from build123d import *

# Parameters (mm, degrees)
SKETCH1_R           = 12.5
BOSS_EXTRUDE1_DEPTH = 17
SKETCH2_R           = 20
BOSS_EXTRUDE2_DEPTH = 26.425
SKETCH3_R           = 12.7
BOSS_EXTRUDE3_DEPTH = 31.75
SKETCH8_W           = 6.35
SKETCH8_H           = 3.175
BOSS_EXTRUDE8_DEPTH = 31.75
SKETCH4_R           = 20
BOSS_EXTRUDE4_DEPTH = 171.45
SKETCH5_R           = 9.525
BOSS_EXTRUDE5_DEPTH = 31.75
SKETCH9_W           = 4.7625
SKETCH9_H           = 2.38125
BOSS_EXTRUDE9_DEPTH = 31.75
SKETCH6_R           = 20
BOSS_EXTRUDE6_DEPTH = 26.425
SKETCH7_R           = 12.5
BOSS_EXTRUDE7_DEPTH = 17


with BuildPart() as part:
    # Sketch1 → Boss-Extrude1 (new body)
    with BuildSketch(Plane(origin=(0, 0, 0), x_dir=(1, 0, 0), z_dir=(0, 1, 0))):
        with Locations(Location((0, 0, 0), (0, 0, 270))):
            Circle(SKETCH1_R)
    extrude(amount=BOSS_EXTRUDE1_DEPTH)

    # Sketch2 → Boss-Extrude2 (add)
    with BuildSketch(Plane(origin=(0, 17, 0), x_dir=(1, 0, 0), z_dir=(0, 1, 0))):
        with Locations(Location((0, 0, 0), (0, 0, 270))):
            Circle(SKETCH2_R)
    extrude(amount=BOSS_EXTRUDE2_DEPTH)

    # Sketch3 → Boss-Extrude3 (add)
    with BuildSketch(Plane(origin=(0, 43.425, 0), x_dir=(1, 0, 0), z_dir=(0, 1, 0))):
        with Locations(Location((0, 0, 0), (0, 0, 270))):
            Circle(SKETCH3_R)
    extrude(amount=BOSS_EXTRUDE3_DEPTH)

    # Sketch8 → Boss-Extrude8 (add)
    with BuildSketch(Plane(origin=(0, 75.175, 0), x_dir=(1, 0, 0), z_dir=(0, 1, 0))):
        with Locations((0, 13.884222124)):
            Rectangle(SKETCH8_W, SKETCH8_H)
    extrude(amount=-BOSS_EXTRUDE8_DEPTH)

    # Sketch4 → Boss-Extrude4 (add)
    with BuildSketch(Plane(origin=(0, 75.175, 0), x_dir=(1, 0, 0), z_dir=(0, 1, 0))):
        with Locations(Location((0, 0, 0), (0, 0, 270))):
            Circle(SKETCH4_R)
    extrude(amount=BOSS_EXTRUDE4_DEPTH)

    # Sketch5 → Boss-Extrude5 (add)
    with BuildSketch(Plane(origin=(0, 246.625, 0), x_dir=(1, 0, 0), z_dir=(0, 1, 0))):
        with Locations(Location((0, 0, 0), (0, 0, 270))):
            Circle(SKETCH5_R)
    extrude(amount=BOSS_EXTRUDE5_DEPTH)

    # Sketch9 → Boss-Extrude9 (add)
    with BuildSketch(Plane(origin=(0, 278.375, 0), x_dir=(1, 0, 0), z_dir=(0, 1, 0))):
        with Locations((0, 10.413166593)):
            Rectangle(SKETCH9_W, SKETCH9_H)
    extrude(amount=-BOSS_EXTRUDE9_DEPTH)

    # Sketch6 → Boss-Extrude6 (add)
    with BuildSketch(Plane(origin=(0, 278.375, 0), x_dir=(1, 0, 0), z_dir=(0, 1, 0))):
        with Locations(Location((0, 0, 0), (0, 0, 270))):
            Circle(SKETCH6_R)
    extrude(amount=BOSS_EXTRUDE6_DEPTH)

    # Sketch7 → Boss-Extrude7 (add)
    with BuildSketch(Plane(origin=(0, 304.8, 0), x_dir=(1, 0, 0), z_dir=(0, 1, 0))):
        with Locations(Location((0, 0, 0), (0, 0, 270))):
            Circle(SKETCH7_R)
    extrude(amount=BOSS_EXTRUDE7_DEPTH)


solid = part.part
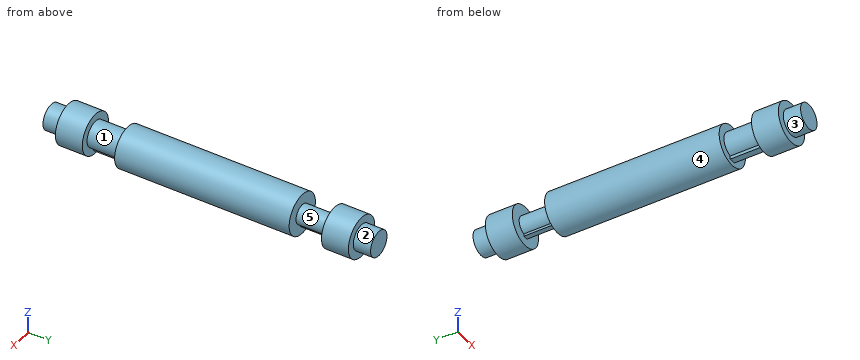
Could you check a few things on this model? Use its own coordinates, in mm. Face numbers are marked on the shaded views. A direction names the side the tool comes from. Coordinates: 2 decimals unless noted, no trailing zeros. Order: outer loops, then holes, each group sorted by start corner. A loop starts at its lowest first (then second) coordinate and runs counter-clockwise, first axis right, second up. Notation, with made-up numbers: (-12, 69) -> (-1, 69) arc R15 ccw to (-1, 86) -> close; hole circle Ø2 at (-29, 19.5). An arc over 180 degrees is marked (long way). One line per question, with ' | ' between items.
Q1. If I drill on L1, parallel to Y at x = -13.5, z = -14 (3 decimals); L2, parallel to Y at x = 4, z = 12 (3 decimals); L3, parallel to Z at x = -2, y = 50.5, over which ranges is the centre line in solid material (lowest first)?
Return value:
L1: 17 to 43.425, 75.175 to 246.625, 278.375 to 304.8 | L2: 17 to 246.625, 278.375 to 304.8 | L3: -15.47 to 12.54
Q2. I'm going to push flat-ended pins straight in: P1, Ø4, axis at x = -1, y = 258, coming from the -Z side; P2, Ø3, axis at x = 15.5, z = 3.5, coming from the -Y side; P3, Ø0.7, axis at y = 262, z = -11, coming from the +X side. Where does each tip first touch, or does it pass through?
Return value:
P1: z = -11.6 | P2: y = 17 | P3: x = 2.38
Q3. On a 3-axis mill with a long thin cutter (end or side, diameter ignored), from which of +Z, -Z, +X, -X, +Y, -Y can I reach the whole of each face in a straight line? I mean the marked faces 3, 4 and 5. Say none if no direction works.
Return value:
face 3: -Y | face 4: +Y, -Y | face 5: none
Q4. Imagine slicing it at A-A on z = 0. Please give me the cut outline in (x, y) (3 decimals), and give its area (3 significant figures).
Return value:
outline: (-20, 17) -> (-12.5, 17) -> (-12.5, 0) -> (12.5, 0) -> (12.5, 17) -> (20, 17) -> (20, 43.425) -> (12.7, 43.425) -> (12.7, 75.175) -> (20, 75.175) -> (20, 246.625) -> (9.525, 246.625) -> (9.525, 278.375) -> (20, 278.375) -> (20, 304.8) -> (12.5, 304.8) -> (12.5, 321.8) -> (-12.5, 321.8) -> (-12.5, 304.8) -> (-20, 304.8) -> (-20, 278.375) -> (-9.525, 278.375) -> (-9.525, 246.625) -> (-20, 246.625) -> (-20, 75.175) -> (-12.7, 75.175) -> (-12.7, 43.425) -> (-20, 43.425) -> close | area: 11,200 mm²
Q5. Thinking about a two-plate mould opening in Y: for the marked faces 1 and 2, which applies, pulls with the +Y half, pulls with the -Y half, needs draft (parallel to the pull), parting line crosses it, or undercut?
Return value:
face 1: undercut | face 2: needs draft
Q6. Imagine slicing it at B-B on x = -6.5. Please give me the cut outline in (y, z) (3 decimals), and give its area (3 significant figures).
Return value:
outline: (0, -10.677) -> (17, -10.677) -> (17, -18.914) -> (43.425, -18.914) -> (43.425, -10.911) -> (75.175, -10.911) -> (75.175, -18.914) -> (246.625, -18.914) -> (246.625, -6.962) -> (278.375, -6.962) -> (278.375, -18.914) -> (304.8, -18.914) -> (304.8, -10.677) -> (321.8, -10.677) -> (321.8, 10.677) -> (304.8, 10.677) -> (304.8, 18.914) -> (278.375, 18.914) -> (278.375, 6.962) -> (246.625, 6.962) -> (246.625, 18.914) -> (75.175, 18.914) -> (75.175, 10.911) -> (43.425, 10.911) -> (43.425, 18.914) -> (17, 18.914) -> (17, 10.677) -> (0, 10.677) -> close | area: 10,300 mm²
Q7. Imagine slicing it at C-C on y = 210. Please give me the cut outline in (x, z), and give its area (3 significant figures).
Return value:
outline: circle Ø40 at (0, 0) | area: 1,260 mm²
